Geometry: final body of the model. Coordinates: model frame, mm. Face numbers are marked on the shaded views. A direction names the side the tool comes from. Give positions to 0.01 mm unless a question says otherwise; leave off trailing zeros. Write each loop counter-clockwise with the first axis right and the second up, starting at its lowest first coordinate (ties: lowest second). Pieces come first, ordered by that corner, then holes.
Q1. Line query: line 1 (X direction, y = 0.6, z = 20); line 2 (X direction, y = 60.25, z = -6); line 3 (Y direction, x = 14.5, z = -2). Output: solid intervals per line, ascending.
Q2. Section B-B (y = 23). Return the cut outline in (x, z).
Q3. Mould query, pull axis Z, two halves, no side actions, for the marked faces 4, 5 and 6. Classes: +Z half, -Z half, draft (parallel to the pull), parting line (faces both ways), or undercut.
Q4. Section A-A (z = 20). Return the cut outline in (x, y).
Q5. Section D-D (y = 38.5). Return the cut outline in (x, z), plus the area to 3 significant figures.
Q6. Reachability of the marked faces 1, 2 and 3 from +Z, -Z, +X, -X, +Y, -Y: full face, straight path, thin tool, end or side. Return the list, or none.
Q7. Pin query (flat end, axial travel): pin 1 Ø5 at (x, z) = (0, 20) entering from -Y; pin 2 Ø11.5 at (x, z) = (0, 0) entering from +Y; pin 3 Ø4 at (x, z) = (17.32, -10) entering from +Y; pin 4 Ø10 at (x, y) = (-7, 31.5) entering from +Z. Return the tip coordinate at first contact, or that it passes through.
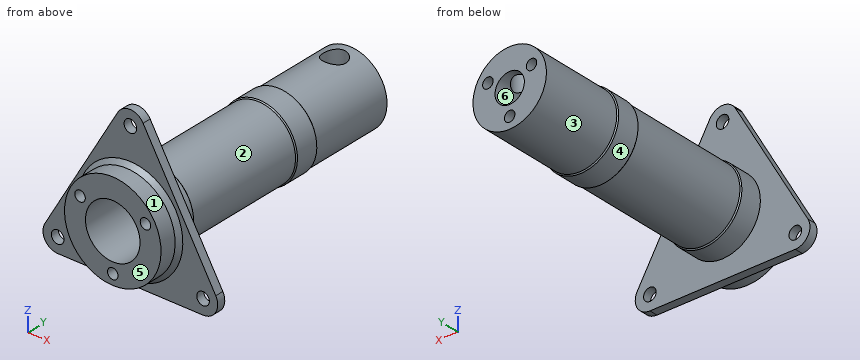
from build123d import *

# Parameters (mm, degrees)
CHAMFER_1_SIZE         = 0.5
CHAMFER_2_SIZE         = 1
SKETCH_9_OUTSIDE_W     = 67.946
SKETCH_9_OUTSIDE_H     = 67.946
SKETCH_9_OUTSIDE_R     = 1.5
CUT_EXTRUDE_2_DEPTH    = 71.786651284
HOLE_WIZARD_M3_1_D     = 2.5
HOLE_WIZARD_M3_1_DEPTH = 5
HOLE_WIZARD_M3_1_TIP   = 0.751075774
HOLE_WIZARD_M3_2_D     = 2.5
HOLE_WIZARD_M3_2_DEPTH = 6.5
HOLE_WIZARD_M3_2_TIP   = 0.751075774
SKETCH_11_R            = 2.75
CUT_EXTRUDE_4_DEPTH    = 70.942787738


with BuildPart() as part:
    # 草图2 → 旋转1 (revolve)
    with BuildSketch(Plane.XY, mode=Mode.PRIVATE) as revolve_1_sk:
        Polygon((9, 2), (9, 7), (8.75, 7), (8.75, 37), (9, 37), (9, 42), (8.75, 42), (8.75, 62.5), (3.5, 62.5), (3.5, 54), (6.5, 51), (6.5, -5), (11.5, -5), (11.5, 0), (23.5, 0), (23.5, 2), align=None)
    revolve(revolve_1_sk.sketch.rotate(Axis((0, 0, 0), (0, 1, 0)), 90), axis=Axis((0, 0, 0), (0, 1, 0)))

    # 倒角1
    # the kernel refuses this chamfer: 0.5 mm, written as the material it adds along each edge
    with BuildSketch(Plane(origin=(0, 42, 0), x_dir=(0, 0, -1), z_dir=(1, 0, 0))) as chamfer_1_piece_1_section:
        Polygon((8.75 + CHAMFER_1_SIZE, 0), (8.75, CHAMFER_1_SIZE), (8.75, 0), align=None)
    chamfer_1_piece_1 = revolve(axis=Axis((0, 42, 0), (0, 1, 0)), mode=Mode.PRIVATE)
    chamfer_1_piece_1 = chamfer_1_piece_1 & Plane(origin=(0, 42.369448451, 0), x_dir=(0, 0, -1), z_dir=(0, 1, 0)) * Cylinder(9, 38, mode=Mode.PRIVATE)
    add(chamfer_1_piece_1)
    with BuildSketch(Plane(origin=(0, 37, 0), x_dir=(0, 0, -1), z_dir=(1, 0, 0))) as chamfer_1_piece_2_section:
        Polygon((8.75, -CHAMFER_1_SIZE), (8.75 + CHAMFER_1_SIZE, 0), (8.75, 0), align=None)
    chamfer_1_piece_2 = revolve(axis=Axis((0, 37, 0), (0, 1, 0)), mode=Mode.PRIVATE)
    chamfer_1_piece_2 = chamfer_1_piece_2 & Plane(origin=(0, 36.630551549, 0), x_dir=(0, 0, -1), z_dir=(0, 1, 0)) * Cylinder(9, 38, mode=Mode.PRIVATE)
    add(chamfer_1_piece_2)
    with BuildSketch(Plane(origin=(0, 7, 0), x_dir=(0, 0, -1), z_dir=(1, 0, 0))) as chamfer_1_piece_3_section:
        Polygon((8.75 + CHAMFER_1_SIZE, 0), (8.75, CHAMFER_1_SIZE), (8.75, 0), align=None)
    chamfer_1_piece_3 = revolve(axis=Axis((0, 7, 0), (0, 1, 0)), mode=Mode.PRIVATE)
    chamfer_1_piece_3 = chamfer_1_piece_3 & Plane(origin=(0, 7.369448451, 0), x_dir=(0, 0, -1), z_dir=(0, 1, 0)) * Cylinder(9, 38, mode=Mode.PRIVATE)
    add(chamfer_1_piece_3)

    # 倒角2
    chamfer_2_edges = [part.edges().sort_by_distance(p)[0] for p in [
        (0, 0, 11.5),
    ]]
    chamfer(chamfer_2_edges, length=CHAMFER_2_SIZE)

    # 草图9 outside → 切除-拉伸2 (cut, through all)
    # profile 1 of 4: a face of its own
    with BuildSketch(Plane.XZ):
        Rectangle(SKETCH_9_OUTSIDE_W, SKETCH_9_OUTSIDE_H)
        with BuildLine():
            Line((-3.031088913, 21.75), (-20.351596989, -8.25))
            ThreePointArc((-20.351596989, -8.25), (-20.351596989, -11.75), (-17.320508076, -13.5))
            Line((-17.320508076, -13.5), (17.320508076, -13.5))
            ThreePointArc((17.320508076, -13.5), (20.351596989, -11.75), (20.351596989, -8.25))
            Line((20.351596989, -8.25), (3.031088913, 21.75))
            ThreePointArc((3.031088913, 21.75), (0, 23.5), (-3.031088913, 21.75))
        make_face(mode=Mode.SUBTRACT)
    # profile 2 of 4: a face of its own
    with BuildSketch(Plane.XZ):
        with Locations(Location((0, 20, 0), (0, 0, 270))):
            Circle(SKETCH_9_OUTSIDE_R)
    # profile 3 of 4: a face of its own
    with BuildSketch(Plane.XZ):
        with Locations(Location((17.320508076, -10, 0), (0, 0, 270))):
            Circle(SKETCH_9_OUTSIDE_R)
    # profile 4 of 4: a face of its own
    with BuildSketch(Plane.XZ):
        with Locations(Location((-17.320508076, -10, 0), (0, 0, 270))):
            Circle(SKETCH_9_OUTSIDE_R)
    extrude(amount=-CUT_EXTRUDE_2_DEPTH, mode=Mode.SUBTRACT)

    # M3 螺纹孔1
    with Locations(Plane.XZ.offset(5)):
        with Locations((0, -9), (7.794228634, 4.5), (-7.794228634, 4.5)):
            Hole(HOLE_WIZARD_M3_1_D / 2, depth=HOLE_WIZARD_M3_1_DEPTH)
            with Locations((0, 0, -(HOLE_WIZARD_M3_1_DEPTH + HOLE_WIZARD_M3_1_TIP / 2))):  # 118° drill point
                Cone(0, HOLE_WIZARD_M3_1_D / 2, HOLE_WIZARD_M3_1_TIP, mode=Mode.SUBTRACT)

    # M3 螺纹孔2
    with Locations(Plane(origin=(0, 62.5, 0), x_dir=(1, 0, 0), z_dir=(0, 1, 0))):
        with Locations((0, 6), (5.196152423, -3), (-5.196152423, -3)):
            Hole(HOLE_WIZARD_M3_2_D / 2, depth=HOLE_WIZARD_M3_2_DEPTH)
            with Locations((0, 0, -(HOLE_WIZARD_M3_2_DEPTH + HOLE_WIZARD_M3_2_TIP / 2))):  # 118° drill point
                Cone(0, HOLE_WIZARD_M3_2_D / 2, HOLE_WIZARD_M3_2_TIP, mode=Mode.SUBTRACT)

    # 草图11 → 切除-拉伸4 (cut, through all)
    with BuildSketch(Plane.XY):
        with Locations(Location((0, 58, 0), (0, 0, 180))):
            Circle(SKETCH_11_R)
    extrude(amount=CUT_EXTRUDE_4_DEPTH, mode=Mode.SUBTRACT)


solid = part.part
Computed:
1. line 1: x = -4.04 to -1.5, 1.5 to 4.04
1. line 2: x = -6.37 to -1.25, 1.25 to 6.37
1. line 3: y = 0 to 2
2. outline: circle Ø17.5 at (0, 0); hole circle Ø13 at (0, 0)
3. face 4: parting line
3. face 5: draft
3. face 6: undercut
4. outline: (-4.04, 0) - (-1.5, 0) - (-1.5, 2) - (-4.04, 2) - close; (1.5, 0) - (4.04, 0) - (4.04, 2) - (1.5, 2) - close
5. outline: circle Ø18 at (0, 0); hole circle Ø13 at (0, 0)
5. area: 122 mm2
6. face 1: -Y
6. face 2: none
6. face 3: +Y
7. pin 1: stops at y = 0
7. pin 2: stops at y = 62.5
7. pin 3: stops at y = 2
7. pin 4: stops at z = 8.52
